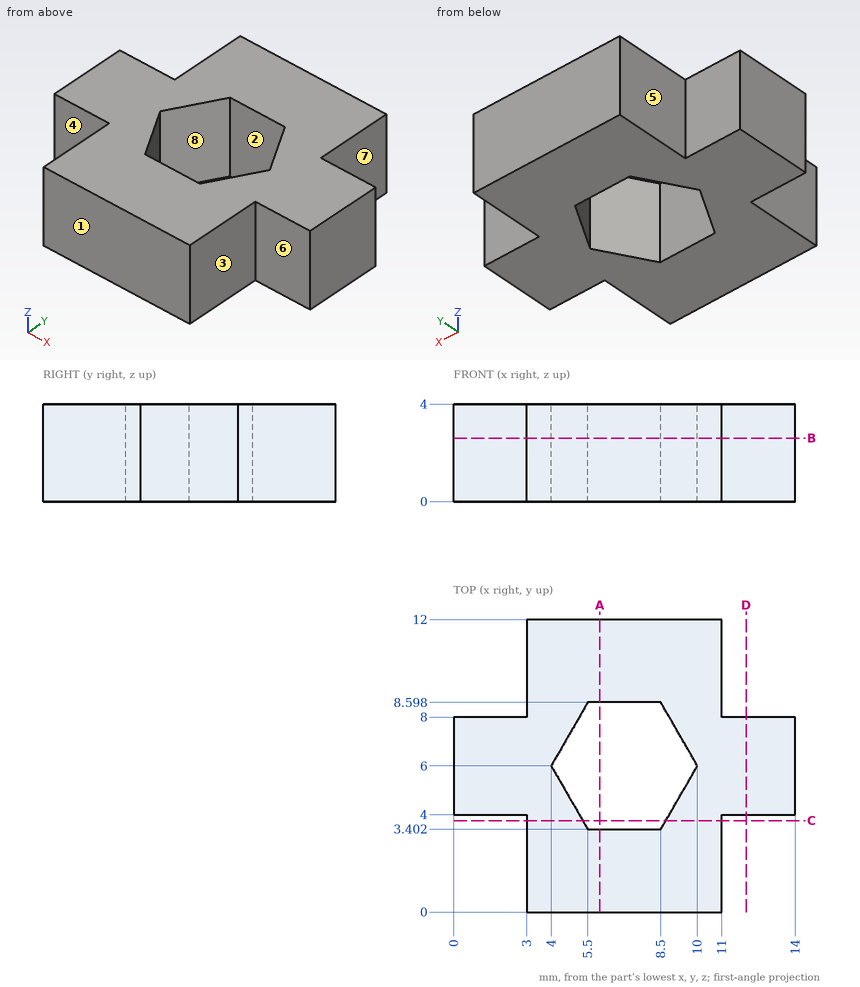
Source: three-view drawing plus pictorial views. Frame: mm from the lowest corner of the part. A direction names the side the tool comes from. Round coordinates to 2 decimals unless told otherwise and drop trailing zeros. Order: outer loops, then holes, each group sorted by start corner. A loop starts at its lowest first (then second) coordinate and runs counter-clockwise, first axis right, second up. Notation, with made-up numbers: (22.5, 80) -> (63.5, 80) arc R23 ccw to (63.5, 118) -> close; hole circle Ø1 at (-2, 80.5). An arc over 180 degrees is marked (long way). Use CSV: the item, a comma, the result in double quotes. Start each with the question number.
1) Section C-C (y = 3.75). Return the cut outline in (x, z).
2) Material intervals for line 1 along Y through (x, z) = (6.75, 1.15); line 2 along X through (y, z) = (2.5, 0.65); line 3 along Y through (x, z) = (2.5, 2.25), sorted ascending. Write a range as from..to.
3) Draft query along Y for the marked faces 1, 2 and 3. Return one class per face: +Y half, -Y half, draft (parallel to the pull), parting line (faces both ways), or undercut.
4) Section D-D (x = 12). Return the cut outline in (y, z).
5) First-contact query: pin 1 Ø2 at (x, y) = (5, 5.5) entering from -Z; pin 2 Ø1.2 at (y, z) = (1, 1.5) entering from -X; pin 3 Ø2 at (y, z) = (2.5, 1) entering from +X; pin 4 Ø0.9 at (x, z) = (2, 2) entering from +Y. Flat tips, straight axial feed; report the tip coordinate or a pass-through.
6) Set-up query: the marked faces 4, 5, 6, 7 and 8. Return all of +Z, -Z, +X, -X, +Y, -Y with unobstructed straight access to the full face (end or side cutting, diameter ignored); none if empty.
7) Section B-B (z = 2.6). Return the cut outline in (x, y), and give its area (3 significant figures).
8) Section A-A (x = 6). Return the cut outline in (y, z), and give its area (3 significant figures).
Returned:
1,outline,"(3, 0) -> (5.3, 0) -> (5.3, 4) -> (3, 4) -> close; (8.7, 0) -> (11, 0) -> (11, 4) -> (8.7, 4) -> close"
2,line 1,"y = 0..3.4, 8.6..12"
2,line 2,"x = 3..11"
2,line 3,"y = 4..8"
3,face 1,"-Y half"
3,face 2,"undercut"
3,face 3,"draft"
4,outline,"(4, 0) -> (8, 0) -> (8, 4) -> (4, 4) -> close"
5,pin 1,"stops at z = 0"
5,pin 2,"stops at x = 3"
5,pin 3,"stops at x = 11"
5,pin 4,"stops at y = 8"
6,face 4,"+Z, -Z, -X, -Y"
6,face 5,"+Z, -Z, -X, +Y"
6,face 6,"+Z, -Z, +X, -Y"
6,face 7,"+Z, -Z, +X, +Y"
6,face 8,"+Z, -Z"
7,outline,"(0, 4) -> (3, 4) -> (3, 0) -> (11, 0) -> (11, 4) -> (14, 4) -> (14, 8) -> (11, 8) -> (11, 12) -> (3, 12) -> (3, 8) -> (0, 8) -> close; hole (4, 6) -> (5.5, 3.4) -> (8.5, 3.4) -> (10, 6) -> (8.5, 8.6) -> (5.5, 8.6) -> close"
7,area,"96.6 mm²"
8,outline,"(0, 0) -> (3.4, 0) -> (3.4, 4) -> (0, 4) -> close; (8.6, 0) -> (12, 0) -> (12, 4) -> (8.6, 4) -> close"
8,area,"27.2 mm²"
